from build123d import *

# Parameters (mm, degrees)
CUT_EXTRUDE_2_DEPTH = 1.5


with BuildPart() as part:
    # 草图1 → 旋转1 (revolve)
    with BuildSketch(Plane(origin=(0, 0, 0), x_dir=(1, 0, 0), z_dir=(0, 1, 0)), mode=Mode.PRIVATE) as revolve_1_sk:
        with BuildLine():
            Line((0, 0), (0, -5.2))
            Line((0, -5.2), (1, -5.2))
            Line((1, -5.2), (1, 0))
            Line((1, 0), (1.8, 0))
            ThreePointArc((1.8, 0), (1.941421356, 0.058578644), (2, 0.2))
            Line((2, 0.2), (2, 0.6))
            ThreePointArc((2, 0.6), (1.941421356, 0.741421356), (1.8, 0.8))
            Line((1.8, 0.8), (0, 0.8))
            Line((0, 0.8), (0, 0))
        make_face()
    revolve(revolve_1_sk.sketch.rotate(Axis((0, 0, 0), (0, 0, 1)), 180), axis=Axis((0, 0, 0), (0, 0, 1)))

    # 草图3 → 切除-拉伸2 (cut)
    with BuildSketch(Plane(origin=(0, 0, -0.8), x_dir=(-1, 0, 0), z_dir=(0, 0, -1))):
        Polygon((0.866025404, 0), (0.433012702, 0.75), (-0.433012702, 0.75), (-0.866025404, 0), (-0.433012702, -0.75), (0.433012702, -0.75), align=None)
    extrude(amount=-CUT_EXTRUDE_2_DEPTH, mode=Mode.SUBTRACT)


solid = part.part
Model file for the job. Use its own axes, mm. A direction names the side the tool comes from. Give positions to 0.01 mm unless a question says otherwise; leave off trailing zeros. Loops run counter-clockwise (first coordinate to the right, second up) from the corner with the lowest first, then second, coordinate; pieces in that order, holes last. Notation, with made-up numbers: (7.25, 16.25) - (18.25, 16.25) arc R35 cw to (18.25, 50.25) - close; hole circle Ø10 at (-39.5, 43). An arc over 180 degrees is marked (long way). Use one line per item in the form item = value.
(1) 3-axis set-ups, long thin cutter, end or side, ignore diameter. For faces 1 (the face through (0, 0, 5.2)), 2 (the face through (0, 0.75, 0)), 3 (the face through (1, 1, 0)): which of +Z, -Z, +X, -X, +Y, -Y reach the whole face in a straight line?
Determined:
face_1 = +Z, +X, -X, +Y, -Y
face_2 = -Z
face_3 = +Z
(2) Cut at B-B (z = -0.3). Give the cut face in (x, y), then the cut area to 3 significant figures.
Determined:
outline = circle Ø4 at (0, 0); hole (-0.87, 0) - (-0.43, -0.75) - (0.43, -0.75) - (0.87, 0) - (0.43, 0.75) - (-0.43, 0.75) - close
area = 10.6 mm^2
(3) Cut at A-A (x = 0). Give the cut face in (y, z).
Determined:
outline = (-2, -0.6) arc R0.2 ccw to (-1.8, -0.8) - (-0.75, -0.8) - (-0.75, 0.7) - (0.75, 0.7) - (0.75, -0.8) - (1.8, -0.8) arc R0.2 ccw to (2, -0.6) - (2, -0.2) arc R0.2 ccw to (1.8, 0) - (1, 0) - (1, 5.2) - (-1, 5.2) - (-1, 0) - (-1.8, 0) arc R0.2 ccw to (-2, -0.2) - close
(4) Cut at C-C (z = 1.85). Give the cut face in (x, y), then the cut area to 3 significant figures.
Determined:
outline = circle Ø2 at (0, 0)
area = 3.14 mm^2
(5) Drill centre lines: L1, parallel to Z at x = 0.15, y = -0.5; L2, parallel to Z at x = -1.45, y = -0.15; L3, parallel to X at y = 0.5, z = 0.25. Where is each one in solid material? Low to high.
Determined:
L1 = 0.7 to 5.2
L2 = -0.8 to 0
L3 = -0.87 to -0.58, 0.58 to 0.87
(6) Pull direction Y, two halves, no side cores. Call faces 4 (the face through (0, 1, -0.8)), 5 (the face through (0, 1, 3)), 6 (the face through (0, 0, 0.7)), 7 (the face through (0, -0.75, 0)): pulls with the +Y half, pulls with the -Y half, needs draft (parallel to the pull), parting line crosses it, or undercut.
Determined:
face_4 = needs draft
face_5 = parting line crosses it
face_6 = undercut
face_7 = undercut
(7) Drop flat-ended pins along their axis: P1, Ø1.5, axis at x = -1, y = -0.5, coming from the +Z side; P2, Ø2, axis at x = 1.5, z = 1.5, coming from the -Y side. Give the stop position or say it passes through.
Determined:
P1 = 5.2
P2 = -0.87
